Here's how the part is built. I have some questions about the finished solid (model axes, mm). A direction names the side the tool comes from. Round coordinates to 2 decimals unless told otherwise and drop trailing zeros. Loops run counter-clockwise (first coordinate to the right, second up) from the corner with the lowest first, then second, coordinate; pieces in that order, holes last. Notation, with made-up numbers: M 55.25,50 L 63.25,50 A9 ccw 63.25,67 Z; hole C 66,14 d8. An arc over 180 degrees is marked long. Answer as CSV lines item,"result".
```python
from build123d import *

# Parameters (mm, degrees)
BOSS_EXTRUDE1_START     = 12.827
BOSS_EXTRUDE1_DEPTH     = 6.35
FILLET1_R               = 6.35
F_1_4_CLEARANCE_HOLE1_D = 7.14248


with BuildPart() as part:
    # Sketch1 → Boss-Extrude1 (new body)
    with BuildSketch(Plane(origin=(0, 144.904574554, 0), x_dir=(-1, 0, 0), z_dir=(0, -1, 0)).offset(BOSS_EXTRUDE1_START)):
        with BuildLine():
            Line((-24.961912484, -1122.100334154), (-9.086912484, -1122.100334154))
            Line((-9.086912484, -1122.100334154), (-9.086912484, -1163.375334154))
            ThreePointArc((-9.086912484, -1163.375334154), (0.438087516, -1172.900334154), (9.963087516, -1163.375334154))
            Line((9.963087516, -1163.375334154), (9.963087516, -1122.100334154))
            Line((9.963087516, -1122.100334154), (25.838087516, -1122.100334154))
            ThreePointArc((25.838087516, -1122.100334154), (35.363087516, -1112.575334154), (25.838087516, -1103.050334154))
            Line((25.838087516, -1103.050334154), (-24.961912484, -1103.050334154))
            ThreePointArc((-24.961912484, -1103.050334154), (-34.486912484, -1112.575334154), (-24.961912484, -1122.100334154))
        make_face()
    extrude(amount=BOSS_EXTRUDE1_DEPTH)

    # Fillet1
    fillet1_edges = [part.edges().sort_by_distance(p)[0] for p in [
        (-9.963087516, 128.902574554, 1122.100334154),
        (9.086912484, 128.902574554, 1122.100334154),
    ]]
    fillet(fillet1_edges, radius=FILLET1_R)

    # 1/4 Clearance Hole1 (through all)
    with Locations(Plane(origin=(0, 125.727574554, 0), x_dir=(-1, 0, 0), z_dir=(0, -1, 0))):
        with Locations((-24.961912484, -1112.575334154), (25.838087516, -1112.575334154), (0.438087516, -1137.975334154), (0.438087516, -1163.375334154), (0.438087516, -1112.575334154)):
            Hole(F_1_4_CLEARANCE_HOLE1_D / 2)


solid = part.part
```
1. We'd pull the mould along X, two halves only. Please class faces 1 (the cylindrical face through (-1.212, 128.947, 1116.062)), 2 (the cylindrical face through (-0.23, 128.95, 1172.9)), 3 (the flat face through (0, 132.078, 1130)), 4 (the cylindrical face through (-1.212, 128.947, 1141.462)): pulls with the +X half, pulls with the -X half, needs draft (parallel to the pull), parting line crosses it, or undercut.
Evaluation:
face 1,"undercut"
face 2,"parting line crosses it"
face 3,"needs draft"
face 4,"undercut"
2. For P1, Ø3, axis at y = 127, z = 1127, coming from the -X side; P2, Ø8, axis at x = -25.84, z = 1112.58, coming from the +Y side; P3, Ø3, axis at y = 128, z = 1162.5, coming from the +X side, each with a flat end and sliding along its axis, tell me the tip position at first contact or that it passes through.
Evaluation:
P1,"stops at x = -10.69"
P2,"stops at y = 132.08"
P3,"stops at x = 9.09"
3. If I drill on line 1 (Z direction, x = 1, y = 127.25); line 2 (Z direction, x = 0, y = 131.75); line 3 (X direction, y = 131.75, z = 1163), over which ranges is the centre line in solid material (lowest first)? Write a range as [from, to].
Evaluation:
line 1,"z = [1103.05, 1109.31], [1115.84, 1134.71], [1141.24, 1160.11], [1166.64, 1172.79]"
line 2,"z = [1103.05, 1109.03], [1116.12, 1134.43], [1141.52, 1159.83], [1166.92, 1172.89]"
line 3,"x = [-9.96, -3.99], [3.11, 9.09]"
4. Which directions (+Z, -Z, +X, -X, +Y, -Y) give clear straight access to the entire face, cutting with the end or side of a thin tool? Please do faces 5 (the cylindrical face through (-26.612, 128.947, 1116.062)), 6 (the flat face through (20, 129, 1122.1)), 7 (the flat face through (-9.963, 129, 1146)).
Evaluation:
face 5,"+Y, -Y"
face 6,"+Z, +X, +Y, -Y"
face 7,"+Z, -X, +Y, -Y"
5. I want a section at B-B, the plane z = 1162. Please give me the cut outline in (x, y).
Evaluation:
outline,"M -9.96,125.73 L -3.73,125.73 L -3.73,132.08 L -9.96,132.08 Z; M 2.86,125.73 L 9.09,125.73 L 9.09,132.08 L 2.86,132.08 Z"
6. I want a section at C-C, the plane y = 128.5. Please give me the cut outline in (x, z) (3 decimals).
Evaluation:
outline,"M -25.838,1103.05 L 24.962,1103.05 A9.525 ccw 24.962,1122.1 L 15.437,1122.1 A6.35 cw 9.087,1128.45 L 9.087,1163.375 A9.525 ccw -9.963,1163.375 L -9.963,1128.45 A6.35 cw -16.313,1122.1 L -25.838,1122.1 A9.525 ccw Z; hole C -25.838,1112.575 d7.142; hole C -0.438,1112.575 d7.142; hole C -0.438,1137.975 d7.142; hole C -0.438,1163.375 d7.142; hole C 24.962,1112.575 d7.142"
7. I want a section at D-D, the plane x = -17.5. Please give me the cut outline in (y, z), and give its area (3 significant figures).
Evaluation:
outline,"M 125.73,1103.05 L 132.08,1103.05 L 132.08,1122.1 L 125.73,1122.1 Z"
area,"121 mm²"
8. I want a section at A-A, the plane z = 1110. Please give me the cut outline in (x, y), and give its area (3 significant figures).
Evaluation:
outline,"M -35.01,125.73 L -28.31,125.73 L -28.31,132.08 L -35.01,132.08 Z; M -23.36,125.73 L -2.91,125.73 L -2.91,132.08 L -23.36,132.08 Z; M 2.04,125.73 L 22.49,125.73 L 22.49,132.08 L 2.04,132.08 Z; M 27.44,125.73 L 34.13,125.73 L 34.13,132.08 L 27.44,132.08 Z"
area,"345 mm²"
